```python
from build123d import *

# Parameters (mm, degrees)
F0_R     = 10
F1_DEPTH = 15


with BuildPart() as f1:
    # F0 (on Front) → F1 (new body, symmetric)
    with BuildSketch(Plane.XZ):
        Polygon((4.132737753, 17.5191460598), (3.1904651552, 17.7149917328), (2.2390718331, 17.8601947729), (1.0773774715, 21.9736036595), (-0.1489718291, 21.9994956168), (-1.4832466893, 17.9387842191), (-2.4399208248, 17.8338662765), (-3.3896198503, 17.6779658691), (-5.7655700937, 21.2310668949), (-6.9398986421, 20.8767288347), (-6.9540406112, 16.6024491921), (-7.8314703545, 16.2070377332), (-8.686511926, 15.7652944965), (-12.044143487, 18.4102853771), (-13.0514998229, 17.7104023775), (-11.7441245865, 13.6409507622), (-12.4564210009, 12.9937514156), (-13.1331076918, 12.3094062552), (-17.1437521993, 13.7873768545), (-17.8855292658, 12.81045834), (-15.3846118211, 9.3441810296), (-15.8620503707, 8.5085461765), (-16.294143373, 7.648587565), (-20.5652109988, 7.8148638232), (-20.9687984885, 6.6565373844), (-17.5191460598, 4.132737753), (-17.7149917328, 3.1904651552), (-17.8601947729, 2.2390718331), (-21.9736036595, 1.0773774715), (-21.9994956168, -0.1489718291), (-17.9387842191, -1.4832466893), (-17.8338662765, -2.4399208248), (-17.6779658691, -3.3896198503), (-21.2310668949, -5.7655700937), (-20.8767288347, -6.9398986421), (-16.6024491921, -6.9540406112), (-16.2070377332, -7.8314703545), (-15.7652944965, -8.686511926), (-18.4102853771, -12.044143487), (-17.7104023775, -13.0514998229), (-13.6409507622, -11.7441245865), (-12.9937514156, -12.4564210009), (-12.3094062552, -13.1331076918), (-13.7873768545, -17.1437521993), (-12.81045834, -17.8855292658), (-9.3441810296, -15.3846118211), (-8.5085461765, -15.8620503707), (-7.648587565, -16.294143373), (-7.8148638232, -20.5652109988), (-6.6565373844, -20.9687984885), (-4.132737753, -17.5191460598), (-3.1904651552, -17.7149917328), (-2.2390718331, -17.8601947729), (-1.0773774715, -21.9736036595), (0.1489718291, -21.9994956168), (1.4832466893, -17.9387842191), (2.4399208248, -17.8338662765), (3.3896198503, -17.6779658691), (5.7655700937, -21.2310668949), (6.9398986421, -20.8767288347), (6.9540406112, -16.6024491921), (7.8314703545, -16.2070377332), (8.686511926, -15.7652944965), (12.044143487, -18.4102853771), (13.0514998229, -17.7104023775), (11.7441245865, -13.6409507622), (12.4564210009, -12.9937514156), (13.1331076918, -12.3094062552), (17.1437521993, -13.7873768545), (17.8855292658, -12.81045834), (15.3846118211, -9.3441810296), (15.8620503707, -8.5085461765), (16.294143373, -7.648587565), (20.5652109988, -7.8148638232), (20.9687984885, -6.6565373844), (17.5191460598, -4.132737753), (17.7149917328, -3.1904651552), (17.8601947729, -2.2390718331), (21.9736036595, -1.0773774715), (21.9994956168, 0.1489718291), (17.9387842191, 1.4832466893), (17.8338662765, 2.4399208248), (17.6779658691, 3.3896198503), (21.2310668949, 5.7655700937), (20.8767288347, 6.9398986421), (16.6024491921, 6.9540406112), (16.2070377332, 7.8314703545), (15.7652944965, 8.686511926), (18.4102853771, 12.044143487), (17.7104023775, 13.0514998229), (13.6409507622, 11.7441245865), (12.9937514156, 12.4564210009), (12.3094062552, 13.1331076918), (13.7873768545, 17.1437521993), (12.81045834, 17.8855292658), (9.3441810296, 15.3846118211), (8.5085461765, 15.8620503707), (7.648587565, 16.294143373), (7.8148638232, 20.5652109988), (6.6565373844, 20.9687984885), align=None)
        Circle(F0_R, mode=Mode.SUBTRACT)
    extrude(amount=F1_DEPTH, both=True)


solid = f1.part
```
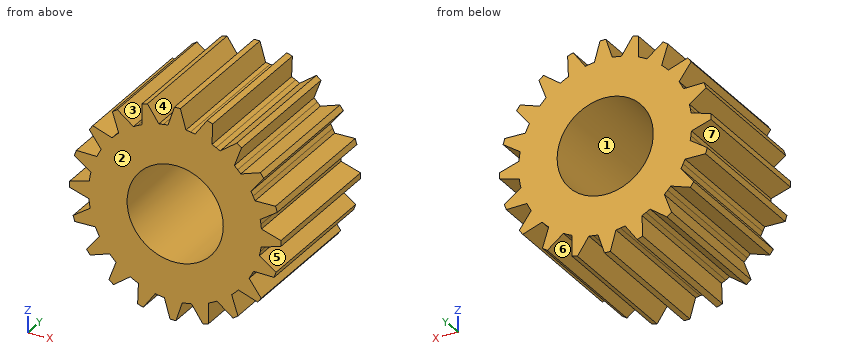
The listing builds one solid part. Answer for the finished solid, in the listing's coordinates (mm). Face numbers are marked on the shaded views. A direction names the side the tool comes from. Coordinates: 2 decimals unless noted, no trailing zeros. Write each loop counter-clockwise with the first axis right and the second up, starting at its lowest first coordinate (ties: lowest second). Pieces come first, ordered by that corner, then holes. Notation, with made-up numbers: (11, 22.25) - (30, 22.25) arc R11 cw to (30, 37.25) - close; hole circle Ø5 at (67.5, 82). An arc over 180 degrees is marked (long way). One line per item, written item: value.
1) Each of these flat-tipped pins is pushed along its axis until it touches: pin 1 Ø2 at (x, y) = (-6, -1.5) entering from +Z; pin 2 Ø2 at (x, y) = (13.5, 5.5) entering from -Z; pin 3 Ø2 at (y, z) = (-9.5, -10) entering from -X. Where does it stop, or does it pass through?
Geometry check:
pin 1: stops at z = 21.23
pin 2: stops at z = -18.09
pin 3: stops at x = -17.59
2) A tool of negligible diameter and unlimited length cuts with its end or side. For the marked faces 4, 5, 6 and 7, from which of +Z, -Z, +X, -X, +Y, -Y can it reach the whole face along a straight path? Write none if from no direction.
Geometry check:
face 4: +Z, +Y, -Y
face 5: +X, +Y, -Y
face 6: -Z, +Y, -Y
face 7: -X, +Y, -Y
3) Find section A-A (x = -11). Give the vertices of the cut face in (y, z).
Geometry check:
outline: (-15, -16.58) - (15, -16.58) - (15, 17.59) - (-15, 17.59) - close
4) Consider line 1 along Z through (x, y) = (0, -5); line 2 along X through (y, z) = (-3, -18) (3 decimals); line 3 along X through (y, z) = (10.75, -4.5). Determine where each line is inside the solid, lowest interval first. Write a range as from..to.
Geometry check:
line 1: z = -22..-10, 10..22
line 2: x = -7.715..-4.485, -2.2..1.463, 3.605..6.949, 11.523..12.635
line 3: x = -19.34..-8.93, 8.93..18.02
5) For a pull along Z with two mould halves and no side action, classify the marked faces 1, 2 and 3 as pulls with the +Z half, pulls with the -Z half, needs draft (parallel to the pull), parting line crosses it, or undercut.
Geometry check:
face 1: undercut
face 2: needs draft
face 3: pulls with the +Z half
